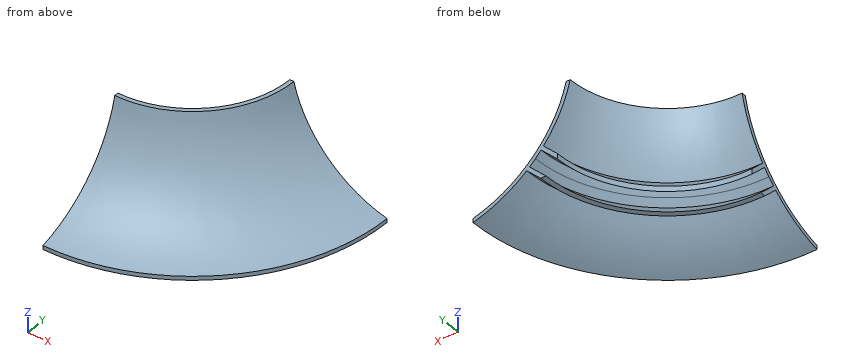
from build123d import *

# Parameters (mm, degrees)
F4_ANGLE = 90


# Not quite as in the source:
# - a feature names something its author has since deleted; it is built from what else it names


with BuildPart() as f4:
    # F1 (on Right) → F4 (revolve)
    with BuildSketch(Plane.YZ):
        with BuildLine():
            Line((-50, 2.0555875069), (-50, 0))
            ThreePointArc((-50, 0), (-35.3898801458, 5.2614268959), (-22.3833982704, 13.7449193584))
            ThreePointArc((-22.3833982704, 13.7449193584), (-21.6521933869, 14.3623617736), (-20.9298823871, 14.9901854251))
            ThreePointArc((-20.9298823871, 14.9901854251), (-19.3758122064, 16.40450242), (-17.8668574762, 17.8668574762))
            ThreePointArc((-17.8668574762, 17.8668574762), (-16.40450242, 19.3758122064), (-14.9901854251, 20.9298823871))
            ThreePointArc((-14.9901854251, 20.9298823871), (-14.3623617736, 21.6521933869), (-13.7449193584, 22.3833982704))
            ThreePointArc((-13.7449193584, 22.3833982704), (-5.2614268959, 35.3898801458), (0, 50))
            Line((0, 50), (-2.0555875069, 50))
            ThreePointArc((-2.0555875069, 50), (-19.2810710386, 19.2810710386), (-50, 2.0555875069))
        make_face()
        with BuildLine():
            ThreePointArc((-20.9298823871, 14.9901854251), (-21.6521933869, 14.3623617736), (-22.3833982704, 13.7449193584))
            Line((-22.3833982704, 13.7449193584), (-15.1433829629, 6.5049040509))
            Line((-15.1433829629, 6.5049040509), (-12.4446010129, 6.5049040509))
            Line((-12.4446010129, 6.5049040509), (-20.9298823871, 14.9901854251))
        make_face()
        with BuildLine():
            ThreePointArc((-13.7449193584, 22.3833982704), (-14.3623617736, 21.6521933869), (-14.9901854251, 20.9298823871))
            Line((-14.9901854251, 20.9298823871), (-6.5049040509, 12.4446010129))
            Line((-6.5049040509, 12.4446010129), (-6.5049040509, 15.1433829629))
            Line((-6.5049040509, 15.1433829629), (-13.7449193584, 22.3833982704))
        make_face()
    revolve(axis=Axis((0, 50, 28.3559039235), (0, 0, 1)), revolution_arc=F4_ANGLE)


solid = f4.part
Verification items for the finished model (mm, model axes). Coordinates: 2 decimals unless noted, no trailing zeros. Order: outer loops, then holes, each group sorted by start corner. A loop starts at its lowest first (then second) coordinate and runs counter-clockwise, first axis right, second up. Notation, with made-up numbers: M -34.5,72 L -6.5,72 A27 ccw -6.5,99 Z; hole C 9.25,75 d11. An arc over 180 degrees is marked long. Return JSON: item names as keys, results as strings.
1) Thickness scan on L1, parallel to X at y = -4, z = 11; L2, parallel to Z at x = 58.5, y = -22; L3, parallel to X at y = 20, z = 33. Record the ranges inside material, lowest first. Write a range as [from, to].
Answer list:
{"L1": "[39.56, 43.97], [53.36, 58.25]", "L2": "[2.12, 4.25]", "L3": "[47.89, 50.58]"}
2) Cross-section at A-A, the plane z = 25. Record the boundary of the cut face in (x, y), and give its area (3 significant figures).
Answer list:
{"outline": "M 0,-14.2 A64.2 ccw 64.2,50 L 61.68,50 A61.68 cw 0,-11.68 Z", "area": "249 mm2"}
3) Gauge pin test, flat ends, axial feed: pin 1 (12 mm diameter, centred on y = -30.5, z = 24, fed in from +X); pin 2 (1 mm diameter, centred on x = 86.5, y = 36, fed in from +Z); pin 3 (12 mm diameter, centred on x = 62.5, y = -1, fed in from +Z); pin 4 (1 mm diameter, centred on x = 80, y = 1.5, fed in from -Z). Record the tip position at first contact, or that the pin passes through.
Answer list:
{"pin 1": "through", "pin 2": "z = 6.64", "pin 3": "z = 14.46", "pin 4": "z = 1.68"}
4) Cross-section at B-B, the plane z = 32.5. Record the boundary of the cut face in (x, y), and give its area (3 significant figures).
Answer list:
{"outline": "M 0,-9.09 A59.09 ccw 59.09,50 L 56.79,50 A56.79 cw 0,-6.79 Z", "area": "210 mm2"}
